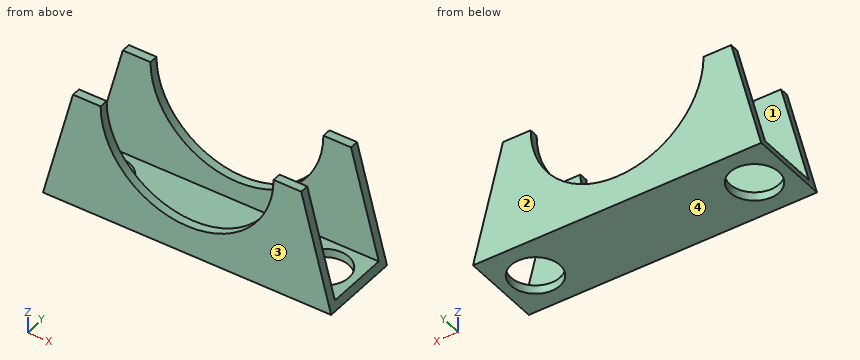
```python
from build123d import *

# Parameters (mm, degrees)
F1_DEPTH = 14
F2_T     = -1.5
F4_D     = 8.5
F5_D     = 8.5


with BuildPart() as f1:
    # F0 (on Front) → F1 (new body)
    with BuildSketch(Plane.XZ):
        with BuildLine():
            Line((-53.882042, 22.777336), (-59.085524, 2.777336))
            Line((-59.085524, 2.777336), (-9.085524, 2.777336))
            Line((-9.085524, 2.777336), (-14.289005, 22.777336))
            Line((-14.289005, 22.777336), (-19.085524, 22.777336))
            ThreePointArc((-19.085524, 22.777336), (-34.085524, 7.777336), (-49.085524, 22.777336))
            Line((-49.085524, 22.777336), (-53.882042, 22.777336))
        make_face()
    extrude(amount=F1_DEPTH)

    # F2
    f2_openings = [f1.faces().sort_by_distance(p)[0] for p in [
        (-56.483783, -7, 12.777336),
        (-51.483783, -7, 22.777336),
        (-34.085524, -7, 7.777336),
        (-16.687264, -7, 22.777336),
        (-11.687264, -7, 12.777336),
    ]]
    offset(amount=F2_T, openings=f2_openings)

    # F4 (through all)
    with Locations(Plane(origin=(0, 0, 2.777336), x_dir=(1, 0, 0), z_dir=(0, 0, -1))):
        with Locations((-53.085524, 7)):
            Hole(F4_D / 2)

    # F5 (through all)
    with Locations(Plane(origin=(0, 0, 2.777336), x_dir=(1, 0, 0), z_dir=(0, 0, -1))):
        with Locations((-15.085524, 7)):
            Hole(F5_D / 2)


solid = f1.part
```
Here's how the part is built. I have some questions about the finished solid (model axes, mm). Face numbers are marked on the shaded views. Give positions to 0.01 mm unless a question says otherwise; leave off trailing zeros. Order: outer loops, then holes, each group sorted by start corner. A loop starts at its lowest first (then second) coordinate and runs counter-clockwise, first axis right, second up. Notation, with made-up numbers: M 60.25,28.25 L 100.25,28.25 A16 cw 100.25,33.25 Z; hole C -2,47 d9. An arc over 180 degrees is marked long. Use a Markdown table: item, result. Add a question column.
1. I need wall thicknesses on probe 1 along Y at (x, z) = (-13.5, 5.25); probe 2 along Z at (x, y) = (-27, -6.25); probe 3 along X at (y, z) = (-6.75, 4). Which ranges of each line are inside material? Lowest first, please. Write a range as from..to.
2. If we mould it in two halves opening along Y, with no side actions, what happens to the marked faces 1, 2, 3 and 4? For each: +Y half, -Y half, draft (parallel to the pull), parting line (faces both ways), or undercut.
3. Suppose I cut it at D-D (y = -3.5). List the corners of the cut face in (x, z) for me.
4. Suppose I cut it at B-B (z = 18.25). List the corners of the cut face in (x, y) for me, and give its area (3 significant figures).
5. For pin 1 Ø3.5 at (x, y) = (-29, -8) entering from +Z; pin 2 Ø8 at (y, z) = (-12, 16) entering from +X; pin 3 Ø4 at (y, z) = (-2.5, 15.5) entering from -X, each with a flat end and sliding along its axis, tell me the tip position at first contact or that it passes through.
6. Suppose I cut it at C-C (x = -52.5). List the corners of the cut face in (y, z) for me, and give its area (3 significant figures).
7. Suppose I cut it at A-A (y = -7). List the corners of the cut face in (x, z) for me, and give its area (3 significant figures).
Results list:
| question | item | result |
|---|---|---|
| 1 | probe 1 | y = -14..-12.5, -1.5..0 |
| 1 | probe 2 | z = 2.78..4.28 |
| 1 | probe 3 | x = -58.77..-57.33, -48.84..-19.33, -10.84..-9.4 |
| 2 | face 1 | undercut |
| 2 | face 2 | +Y half |
| 2 | face 3 | -Y half |
| 2 | face 4 | draft |
| 3 | outline | M -59.09,2.78 L -55.5,2.78 L -55.5,4.28 L -58.7,4.28 Z; M -50.67,2.78 L -17.5,2.78 L -17.5,4.28 L -50.67,4.28 Z; M -12.67,2.78 L -9.09,2.78 L -9.48,4.28 L -12.67,4.28 Z |
| 4 | outline | M -55.06,-14 L -48.39,-14 L -48.39,-12.5 L -55.06,-12.5 Z; M -55.06,-1.5 L -48.39,-1.5 L -48.39,0 L -55.06,0 Z; M -19.79,-14 L -13.11,-14 L -13.11,-12.5 L -19.79,-12.5 Z; M -19.79,-1.5 L -13.11,-1.5 L -13.11,0 L -19.79,0 Z |
| 4 | area | 40.0 mm² |
| 5 | pin 1 | stops at z = 4.28 |
| 5 | pin 2 | stops at x = -11.49 |
| 5 | pin 3 | stops at x = -56.23 |
| 6 | outline | M -14,2.78 L -11.21,2.78 L -11.21,4.28 L -12.5,4.28 L -12.5,22.78 L -14,22.78 Z; M -2.79,2.78 L 0,2.78 L 0,22.78 L -1.5,22.78 L -1.5,4.28 L -2.79,4.28 Z |
| 6 | area | 63.9 mm² |
| 7 | outline | M -59.09,2.78 L -57.34,2.78 L -57.34,4.28 L -58.7,4.28 Z; M -48.84,2.78 L -19.34,2.78 L -19.34,4.28 L -48.84,4.28 Z; M -10.84,2.78 L -9.09,2.78 L -9.48,4.28 L -10.84,4.28 Z |
| 7 | area | 48.9 mm² |
